Build history of the part. All positions in model axes, mm. Face numbers are marked on the shaded views. Round coordinates to 2 decimals unless told otherwise and drop trailing zeros. Write each loop counter-clockwise with the first axis right and the second up, starting at its lowest first coordinate (ties: lowest second). Pieces come first, ordered by that corner, then holes. Notation, with made-up numbers: (68, 61.25) - (104, 61.25) arc R25 cw to (104, 80.25) - close; hole circle Ø11 at (12, -2). An arc over 180 degrees is marked (long way). One line per question, with ' | ' between items.
from build123d import *

# Parameters (mm, degrees)
F0_W     = 9
F0_H     = 9
F1_DEPTH = 25
F3_DEPTH = 9
F4_R     = 4
F4_R_2   = 2
F5_DEPTH = 4
F6_DEPTH = 162.001
F7_R     = 5
F8_R     = 5
F9_R     = 5
F10_R    = 5
F11_R    = 3
F12_R    = 3


with BuildPart() as f1:
    # F0 (on Top) → F1 (new body)
    with BuildSketch(Plane.XY):
        Polygon((-148.6704205513, 24.2638568878), (-148.6704205513, 15.2638568878), (-84.8983426127, 15.2638568878), (-72.1704205513, 15.2638568878), (4.3295794487, 15.2638568878), (4.3295794487, 24.2638568878), align=None)
        with Locations((-153.1704205513, 19.7638568878)):
            Rectangle(F0_W, F0_H)
        Polygon((-148.6704205513, -48.5082210508), (-148.6704205513, 15.2638568878), (-157.6704205513, 15.2638568878), (-157.6704205513, -61.2361431122), (-148.6704205513, -61.2361431122), align=None)
        Polygon((-72.1704205513, 15.2638568878), (-84.8983426127, 15.2638568878), (-116.784381582, -16.6221820815), (-110.4204205513, -22.9861431122), align=None)
        with Locations((-153.1704205513, 28.7638568878)):
            Rectangle(F0_W, F0_H)
        Polygon((-116.784381582, -16.6221820815), (-148.6704205513, -48.5082210508), (-148.6704205513, -61.2361431122), (-110.4204205513, -22.9861431122), align=None)
        Polygon((4.3295794487, 33.2638568878), (4.3295794487, 24.2638568878), (4.3295794487, 15.2638568878), (13.3295794487, 15.2638568878), (13.3295794487, 33.2638568878), align=None)
    extrude(amount=F1_DEPTH)

    # F2 (on face) → F3 (cut, through all)
    with BuildSketch(Plane(origin=(-157.6704205513, 0, 0), x_dir=(0, -1, 0), z_dir=(-1, 0, 0))):
        with BuildLine():
            ThreePointArc((-3.2638568878, 12.5), (-5.2638568878, 14.5), (-7.2638568878, 12.5))
            Line((-7.2638568878, 12.5), (-3.2638568878, 12.5))
        make_face()
        with BuildLine():
            Line((-3.2638568878, 12.5), (-7.2638568878, 12.5))
            ThreePointArc((-7.2638568878, 12.5), (-5.2638568878, 10.5), (-3.2638568878, 12.5))
        make_face()
        with BuildLine():
            ThreePointArc((32.7361431122, 12.5), (34.7361431122, 10.5), (36.7361431122, 12.5))
            Line((36.7361431122, 12.5), (32.7361431122, 12.5))
        make_face()
        with BuildLine():
            Line((32.7361431122, 12.5), (36.7361431122, 12.5))
            ThreePointArc((36.7361431122, 12.5), (34.7361431122, 14.5), (32.7361431122, 12.5))
        make_face()
    extrude(amount=-F3_DEPTH, mode=Mode.SUBTRACT)

    # F4 (on face) → F5 (cut)
    with BuildSketch(Plane.YZ.offset(-148.6704205513)):
        with Locations((5.2638568876, 12.5)):
            Circle(F4_R)
        with Locations((5.2638568878, 12.5)):
            Circle(F4_R_2, mode=Mode.SUBTRACT)
        with Locations((-34.7361431124, 12.5)):
            Circle(F4_R)
        with Locations((-34.7361431122, 12.5)):
            Circle(F4_R_2, mode=Mode.SUBTRACT)
    extrude(amount=-F5_DEPTH, mode=Mode.SUBTRACT)

    # F4 (on face) → F6 (cut, through all)
    with BuildSketch(Plane.YZ.offset(-148.6704205513)):
        with Locations((-34.7361431124, 12.5)):
            Circle(F4_R)
        with Locations((-34.7361431122, 12.5)):
            Circle(F4_R_2, mode=Mode.SUBTRACT)
        with Locations((-34.7361431122, 12.5)):
            Circle(F4_R_2)
    extrude(amount=F6_DEPTH, mode=Mode.SUBTRACT)

    # F7
    f7_edges = [f1.edges().sort_by_distance(p)[0] for p in [
        (-148.670421, -61.236143, 12.5),
    ]]
    fillet(f7_edges, radius=F7_R)

    # F8
    f8_edges = [f1.edges().sort_by_distance(p)[0] for p in [
        (-72.170421, 15.263857, 12.5),
    ]]
    fillet(f8_edges, radius=F8_R)

    # F9
    f9_edges = [f1.edges().sort_by_distance(p)[0] for p in [
        (13.329579, 15.263857, 12.5),
    ]]
    fillet(f9_edges, radius=F9_R)

    # F10
    f10_edges = [f1.edges().sort_by_distance(p)[0] for p in [
        (13.329579, 33.263857, 12.5),
    ]]
    fillet(f10_edges, radius=F10_R)

    # F11
    f11_edges = [f1.edges().sort_by_distance(p)[0] for p in [
        (-157.670421, 33.263857, 12.5),
        (-116.784382, 15.263857, 25),
        (-30.884887, 15.263857, 25),
        (-116.784382, -16.622182, 25),
        (-148.670421, -16.622182, 25),
        (-72.170421, 24.263857, 25),
    ]]
    fillet(f11_edges, radius=F11_R)

    # F12
    f12_edges = [f1.edges().sort_by_distance(p)[0] for p in [
        (-116.784382, 15.263857, 0),
        (-30.884887, 15.263857, 0),
        (-110.420421, -22.986143, 0),
        (-116.784382, -16.622182, 0),
        (-148.670421, -16.622182, 0),
        (-72.170421, 24.263857, 0),
    ]]
    fillet(f12_edges, radius=F12_R)


solid = f1.part
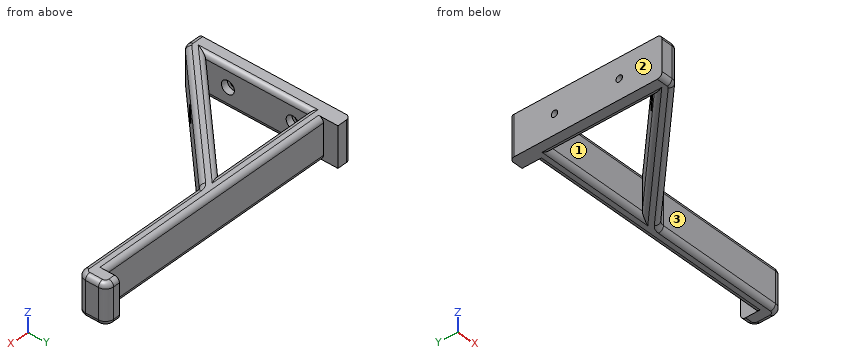
Q1. Saw through at B-B, the plane x = -46.5. List the corners of the cut face in (y, z).
Found:
outline: (15.26, 3) arc R3 ccw to (18.26, 0) - (21.26, 0) arc R3 ccw to (24.26, 3) - (24.26, 22) arc R3 ccw to (21.26, 25) - (18.26, 25) arc R3 ccw to (15.26, 22) - close
Q2. Saw through at A-A, the plane z = 6. List the corners of the cut face in (x, y).
Found:
outline: (-157.67, -61.24) - (-150.74, -61.24) arc R5 ccw to (-147.21, -59.77) - (-73.63, 13.8) arc R5 cw to (-70.1, 15.26) - (8.33, 15.26) arc R5 ccw to (13.33, 20.26) - (13.33, 28.26) arc R5 ccw to (8.33, 33.26) - (4.33, 33.26) - (4.33, 24.26) - (-148.67, 24.26) - (-148.67, 33.26) - (-154.67, 33.26) arc R3 ccw to (-157.67, 30.26) - close; hole (-148.67, -48.51) - (-84.9, 15.26) - (-148.67, 15.26) - close
Q3. Drill centre lines: L1, parallel to Y at x = -154.5, z = 12.5; L2, parallel to Y at x = -67, z = 20; L3, parallel to Y at x = -128, z = 15.25. Where is each one in solid material? Low to high. Write a range as from..to.
Found:
L1: -61.24..-36.74, -32.74..3.26, 7.26..33.26 | L2: 15.26..24.26 | L3: -40.57..-37.64, -31.83..-27.84, 15.26..24.26
Q4. Drop flat-ended pins along their axis: pin 1 (10.5 mm diameter, centred on y = -34.74, z = 12.5, fed in from +X); pin 2 (5 mm diameter, centred on y = -34.74, z = 12.5, fed in from -X); pin 3 (10 mm diameter, centred on x = -131, z = 19.5, fed in from +Y); pin 4 (1 mm diameter, centred on y = 8.5, z = 7, fed in from +X). Give the stop position or say it passes through.
Found:
pin 1: x = -116.92 | pin 2: x = -157.67 | pin 3: y = 24.26 | pin 4: x = -78.43
Q5. Pull direction X, two halves, no side cores. Call the marked faces 1, 2 and 3: +X half, -X half, draft (parallel to the pull), parting line (faces both ways), or undercut.
Found:
face 1: undercut | face 2: -X half | face 3: draft
